Could you check a few things on this model? Use its own coordinates, in mm. A direction names the side the tool comes from. Coordinates: 2 decimals unless noted, no trailing zeros. Loops run counter-clockwise (first coordinate to the right, second up) from the corner with the lowest first, then second, coordinate; pieces in that order, holes last.
from build123d import *
from build123d.topology import SkipClean

# Parameters (mm, degrees)
SKETCH1_R                      = 137.5
BOSS_EXTRUDE1_DEPTH            = 6.25
BOSS_EXTRUDE2_START            = 162.5
BOSS_EXTRUDE2_DEPTH            = 162.5
BOSS_EXTRUDE3_START            = 12.5
SKETCH3_R                      = 137.5
BOSS_EXTRUDE3_DEPTH            = 12.5
SKETCH4_R                      = 37.5
BOSS_EXTRUDE4_DEPTH            = 62.5
CUT_EXTRUDE1_REACH             = 313.812
SKETCH5_R                      = 18.75
CUT_EXTRUDE1_DIRECTION_2_DEPTH = 312.811742082
SKETCH6_R                      = 100
CUT_EXTRUDE2_DEPTH             = 6.25


with BuildPart() as part:
    # Sketch1 → Boss-Extrude1 (new body)
    with BuildSketch(Plane(origin=(0, 0, 0), x_dir=(1, 0, 0), z_dir=(0, 1, 0))):
        with Locations(Location((0, 0, 0), (0, 0, 270))):
            Circle(SKETCH1_R)
    extrude(amount=BOSS_EXTRUDE1_DEPTH)

    # Sketch2 → Boss-Extrude2 (add)
    with SkipClean():  # the faces are left unmerged after this step: merging them gives an invalid solid
        with BuildSketch(Plane.XZ.offset(BOSS_EXTRUDE2_START)):
            with BuildLine():
                Line((137.5, 0), (75.5, 0))
                Line((75.5, 0), (75.5, -6.25))
                Line((75.5, -6.25), (133.603892159, -6.25))
                ThreePointArc((133.603892159, -6.25), (132.161525003, -20.552221504), (129.192579266, -34.617047282))
                Line((129.192579266, -34.617047282), (132.814801115, -35.587618702))
                ThreePointArc((132.814801115, -35.587618702), (136.323668439, -17.94735143), (137.5, 0))
            make_face()
            with BuildLine():
                Line((68.75, -119.07849302), (37.75, -65.384917986))
                Line((37.75, -65.384917986), (32.337341226, -68.509917986))
                Line((32.337341226, -68.509917986), (61.389287306, -118.829364654))
                ThreePointArc((61.389287306, -118.829364654), (48.282016575, -124.731348808), (34.617047282, -129.192579266))
                Line((34.617047282, -129.192579266), (35.587618702, -132.814801115))
                ThreePointArc((35.587618702, -132.814801115), (52.61897195, -127.03343572), (68.75, -119.07849302))
            make_face()
            with BuildLine():
                Line((-68.75, -119.07849302), (-37.75, -65.384917986))
                Line((-37.75, -65.384917986), (-43.162658774, -62.259917986))
                Line((-43.162658774, -62.259917986), (-72.214604853, -112.579364654))
                ThreePointArc((-72.214604853, -112.579364654), (-83.879508429, -104.179127304), (-94.575531984, -94.575531984))
                Line((-94.575531984, -94.575531984), (-97.227182413, -97.227182413))
                ThreePointArc((-97.227182413, -97.227182413), (-83.704696489, -109.08608429), (-68.75, -119.07849302))
            make_face()
            with BuildLine():
                Line((-137.5, 0), (-75.5, 0))
                Line((-75.5, 0), (-75.5, 6.25))
                Line((-75.5, 6.25), (-133.603892159, 6.25))
                ThreePointArc((-133.603892159, 6.25), (-132.161525003, 20.552221504), (-129.192579266, 34.617047282))
                Line((-129.192579266, 34.617047282), (-132.814801115, 35.587618702))
                ThreePointArc((-132.814801115, 35.587618702), (-136.323668439, 17.94735143), (-137.5, 0))
            make_face()
            with BuildLine():
                Line((-68.75, 119.07849302), (-37.75, 65.384917986))
                Line((-37.75, 65.384917986), (-32.337341226, 68.509917986))
                Line((-32.337341226, 68.509917986), (-61.389287306, 118.829364654))
                ThreePointArc((-61.389287306, 118.829364654), (-48.282016575, 124.731348808), (-34.617047282, 129.192579266))
                Line((-34.617047282, 129.192579266), (-35.587618702, 132.814801115))
                ThreePointArc((-35.587618702, 132.814801115), (-52.61897195, 127.03343572), (-68.75, 119.07849302))
            make_face()
            with BuildLine():
                Line((68.75, 119.07849302), (37.75, 65.384917986))
                Line((37.75, 65.384917986), (43.162658774, 62.259917986))
                Line((43.162658774, 62.259917986), (72.214604853, 112.579364654))
                ThreePointArc((72.214604853, 112.579364654), (83.879508429, 104.179127304), (94.575531984, 94.575531984))
                Line((94.575531984, 94.575531984), (97.227182413, 97.227182413))
                ThreePointArc((97.227182413, 97.227182413), (83.704696489, 109.08608429), (68.75, 119.07849302))
            make_face()
        extrude(amount=-BOSS_EXTRUDE2_DEPTH)

    # Sketch3 → Boss-Extrude3 (add)
    with BuildSketch(Plane.XZ.offset(162.5).offset(BOSS_EXTRUDE3_START)):
        with Locations(Location((0, 0, 0), (0, 0, 270))):
            Circle(SKETCH3_R)
    extrude(amount=-BOSS_EXTRUDE3_DEPTH)

    # Sketch4 → Boss-Extrude4 (add)
    with BuildSketch(Plane.XZ.offset(175)):
        with Locations(Location((0, 0, 0), (0, 0, 270))):
            Circle(SKETCH4_R)
    extrude(amount=BOSS_EXTRUDE4_DEPTH)

    # Sketch5 → Cut-Extrude1 (cut, up to next)
    with BuildSketch(Plane.XZ.offset(237.5), mode=Mode.PRIVATE) as cut_extrude1_sk1:
        with Locations(Location((0, 0, 0), (0, 0, 90))):
            Circle(SKETCH5_R)
    cut_extrude1_tool1 = extrude(cut_extrude1_sk1.sketch, amount=-CUT_EXTRUDE1_REACH, mode=Mode.PRIVATE) & part.part
    add(cut_extrude1_tool1.solids().sort_by_distance((0, -237.5, 0))[0], mode=Mode.SUBTRACT)

    # Sketch5 → Cut-Extrude1 direction 2 (cut)
    with BuildSketch(Plane.XZ.offset(237.5)):
        with Locations(Location((0, 0, 0), (0, 0, 90))):
            Circle(SKETCH5_R)
    extrude(amount=CUT_EXTRUDE1_DIRECTION_2_DEPTH, mode=Mode.SUBTRACT)

    # Sketch6 → Cut-Extrude2 (cut)
    with BuildSketch(Plane(origin=(0, 6.25, 0), x_dir=(1, 0, 0), z_dir=(0, 1, 0))):
        with Locations(Location((0, 0, 0), (0, 0, 270))):
            Circle(SKETCH6_R)
    extrude(amount=-CUT_EXTRUDE2_DEPTH, mode=Mode.SUBTRACT)


solid = part.part
1) Imagine slicing it at B-B on z = 57.5. List the corners of the cut face in (x, y) for me, plus the area to 3 significant figures.
2) If I drill on L1, parallel to Y at x = 59, z = 89; L2, parallel to X at y = 4.5, z = 0; L3, parallel to X at y = -179, z = 0, over which ranges is the centre line in solid material (lowest first)?
3) We'd pull the mould along Y, two halves only. Please class faces 6 (the flat face through (-53.47, -82.39, -92.61)), 7 (the flat face through (-29, -175, -29)), 8 (the flat face through (47, 0, 74)), 9 (the flat face through (5, 0, 112)): released by +Y, released by -Y, zero draft, split by the parting line, or undercut.
4) For faces 1 (the cylindrical face through (132.192, -82.388, -20.353)), 2 (the flat face through (107, -82, 0)), 3 (the flat face through (-57.485, -82.388, -87.067)), 4 (the flat face through (41, 0, -78)), 5 (the flat face through (-101, 6.25, 10)), which set-ups out of +Z, -Z, +X, -X, +Y, -Y let a thin tool reach every point of the face, with its end or its side?
5) Imagine slicing it at A-A on x = 0. List the corners of the cut face in (y, z) for me, plus the area to 3 significant figures.
6) Imagine slicing it at C-C on y = -100. State how many separate pieces and enclosed holes the cut face has, plus the area to 3 significant figures.
7) Imagine slicing it at D-D on x = -88. List the corners of the cut face in (y, z) for me.
8) Will these pins go through, and if not, where does the flat tip stop? pin 1 (7 mm diameter, centred on x = -88.5, z = 4.5, fed in from +Y); pin 2 (18.5 mm diameter, centred on x = -93, y = -119.5, fed in from -Z); pin 3 (1.5 mm diameter, centred on x = -82.5, y = -149, fed in from -Z).
Solved:
1. outline: (-124.9, -175) - (124.9, -175) - (124.9, -162.5) - (-124.9, -162.5) - close; (-124.9, 0) - (-81.82, 0) - (-81.82, 6.25) - (-124.9, 6.25) - close; (81.82, 0) - (124.9, 0) - (124.9, 6.25) - (81.82, 6.25) - close
1. area: 3,660 mm2
2. L1: y = -175 to -162.5, 0 to 6.25
2. L2: x = -137.5 to -100, 100 to 137.5
2. L3: x = -37.5 to -18.75, 18.75 to 37.5
3. face 6: undercut
3. face 7: released by -Y
3. face 8: released by +Y
3. face 9: undercut
4. face 1: -X
4. face 2: +X
4. face 3: none
4. face 4: +Y
4. face 5: +Z, -Z, +X, -X, +Y
5. outline: (-237.5, -37.5) - (-175, -37.5) - (-175, -137.5) - (-162.5, -137.5) - (-162.5, -18.75) - (-237.5, -18.75) - close; (-237.5, 18.75) - (-162.5, 18.75) - (-162.5, 137.5) - (-175, 137.5) - (-175, 37.5) - (-237.5, 37.5) - close; (0, -137.5) - (6.25, -137.5) - (6.25, -100) - (0, -100) - close; (0, 100) - (6.25, 100) - (6.25, 137.5) - (0, 137.5) - close
5. area: 5,780 mm2
6. separate pieces: 6
6. enclosed holes: 0
6. area: 2,980 mm2
7. outline: (-175, -105.65) - (6.25, -105.65) - (6.25, -47.5) - (0, -47.5) - (0, -100.72) - (-162.5, -100.72) - (-162.5, 0) - (0, 0) - (0, 6.25) - (-162.5, 6.25) - (-162.5, 105.65) - (-175, 105.65) - close; (0, 47.5) - (6.25, 47.5) - (6.25, 105.65) - (0, 105.65) - close
8. pin 1: stops at y = 0
8. pin 2: stops at z = -109.05
8. pin 3: stops at z = -110.56
